Can you work these out from the model? Positions are in its coordinate system, mm. Coordinates: 2 decimals unless noted, no trailing zeros. Order: outer loops, then holes, each group sorted by start corner. A loop starts at its lowest first (then second) coordinate and runs counter-clockwise, first axis right, second up. Notation, with made-up numbers: (5, -22.75) -> (52, -22.75) arc R24 cw to (52, -12.75) -> close; hole circle Ø5 at (35.25, -19.5). An arc over 180 degrees is marked (long way). Answer as a JSON object with one key per item and string values. Group by question number.
(1) I need wall thicknesses on line 1 (X direction, y = 0.3, z = -119.5); line 2 (X direction, y = -1.2, z = 246); line 3 (Y direction, x = 4.5, z = 83.5). Which ranges of each line are inside material? Lowest first, please.
(2) I want a section at B-B, the plane z = 90.5. List the corners of the cut face in (x, y) for me, plus the area to 3 significant figures.
(3) I want a section at A-A, the plane y = -1.6. List the corners of the cut face in (x, z) for me.
(4) For pin 1 (13.5 mm diameter, centred on x = -9, z = 228.5, fed in from -Y); pin 2 (7.5 mm diameter, centred on x = 0, z = 254.5, fed in from +Y), each with a flat end and sliding along its axis, tell me the tip position at first contact or that it passes through.
from build123d import *

# Parameters (mm, degrees)
SKETCH1_W           = 25
SKETCH1_H           = 5.8
EXTRUDE1_DEPTH      = 259.4
SKETCH6_W           = 25
SKETCH6_H           = 20
BOSS_EXTRUDE2_DEPTH = 5.8
CUT_EXTRUDE2_DEPTH  = 559.8
SKETCH8_W           = 88.25
SKETCH8_H           = 0.06858
CUT_EXTRUDE3_DEPTH  = 26


with BuildPart() as part:
    # Sketch1 → Extrude1 (new body, symmetric)
    with BuildSketch(Plane.XY):
        Rectangle(SKETCH1_W, SKETCH1_H)
    extrude(amount=EXTRUDE1_DEPTH, both=True)

    # Sketch6 → Boss-Extrude2 (add)
    with BuildSketch(Plane(origin=(0, 2.9, 0), x_dir=(1, 0, 0), z_dir=(0, 1, 0))):
        with Locations((0, 269.4)):
            Rectangle(SKETCH6_W, SKETCH6_H)
        with Locations((0, -269.4)):
            Rectangle(SKETCH6_W, SKETCH6_H)
    extrude(amount=-BOSS_EXTRUDE2_DEPTH)

    # Sketch7 → Cut-Extrude2 (cut, through all)
    with BuildSketch(Plane.XY.offset(279.4)):
        with BuildLine():
            Line((-0.00025, 0.0222), (-0.00025, -2.9))
            Line((-0.00025, -2.9), (4.76225, -2.9))
            Line((4.76225, -2.9), (4.76225, 0.0222))
            ThreePointArc((4.76225, 0.0222), (2.381, 2.40345), (-0.00025, 0.0222))
        make_face()
    extrude(amount=-CUT_EXTRUDE2_DEPTH, mode=Mode.SUBTRACT)

    # Sketch8 → Cut-Extrude3 (cut, through all)
    with BuildSketch(Plane.ZY.offset(12.5)):
        with Locations((235.275, 2.86571)):
            Rectangle(SKETCH8_W, SKETCH8_H)
        with Locations((235.275, -2.86571)):
            Rectangle(SKETCH8_W, SKETCH8_H)
    extrude(amount=-CUT_EXTRUDE3_DEPTH, mode=Mode.SUBTRACT)


solid = part.part
Computed values:
{
 "1": {"line 1": "x = -12.5 to 0.02, 4.75 to 12.5", "line 2": "x = -12.5 to 0, 4.76 to 12.5", "line 3": "y = 1.11 to 2.9"},
 "2": {"outline": "(-12.5, -2.9) -> (0, -2.9) -> (0, 0.02) arc R2.38 cw to (4.76, 0.02) -> (4.76, -2.9) -> (12.5, -2.9) -> (12.5, 2.9) -> (-12.5, 2.9) -> close", "area": "122 mm2"},
 "3": {"outline": "(-12.5, -279.4) -> (0, -279.4) -> (0, 279.4) -> (-12.5, 279.4) -> close; (4.76, -279.4) -> (12.5, -279.4) -> (12.5, 279.4) -> (4.76, 279.4) -> close"},
 "4": {"pin 1": "stops at y = -2.83", "pin 2": "stops at y = 2.83"}
}
